Build history of the part. All positions in model axes, mm. Face numbers are marked on the shaded views. A direction names the side the tool comes from. Give positions to 0.01 mm unless a question says otherwise; leave off trailing zeros. Order: outer loops, then holes, each group sorted by start corner. A loop starts at its lowest first (then second) coordinate and runs counter-clockwise, first axis right, second up. Notation, with made-up numbers: (-0.75, 81) - (49.25, 81) arc R21 ccw to (49.25, 120) - close; hole circle Ø10 at (63, 63). An arc over 180 degrees is marked (long way). One line per item, written item: value.
```python
from build123d import *

# Parameters (mm, degrees)
F1_DEPTH = 50.8
F2_W     = 50.8
F2_H     = 127
F3_DEPTH = 76.2
F4_W     = 50.8
F4_H     = 25.4
F5_DEPTH = 25.4


with BuildPart() as f1:
    # F0 (on Front) → F1 (new body)
    with BuildSketch(Plane.XZ):
        Polygon((100.034788, 58.857108), (-103.165212, 58.857108), (-103.165212, -68.142892), (100.034788, -68.142892), (100.034788, -30.042892), (-1.565212, -30.042892), (-1.565212, 20.757108), (100.034788, 20.757108), align=None)
    extrude(amount=F1_DEPTH)

    # F2 (on face) → F3 (join)
    with BuildSketch(Plane(origin=(0, 0, 0), x_dir=(-1, 0, 0), z_dir=(0, 1, 0))):
        with Locations((77.765212, -4.642892)):
            Rectangle(F2_W, F2_H)
    extrude(amount=F3_DEPTH)

    # F4 (on face) → F5 (join)
    with BuildSketch(Plane(origin=(0, 76.2, 0), x_dir=(-1, 0, 0), z_dir=(0, 1, 0))):
        with Locations((77.765212, 46.157108)):
            Rectangle(F4_W, F4_H)
        with Locations((77.765212, -55.442892)):
            Rectangle(F4_W, F4_H)
    extrude(amount=F5_DEPTH)


solid = f1.part
```
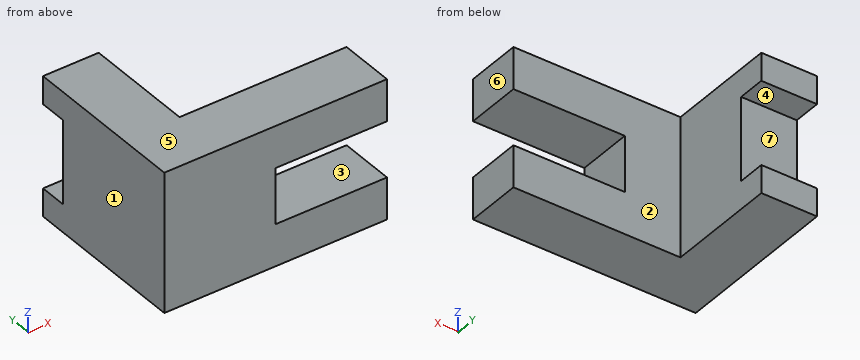
(1) Slice it at C-C, the plane z = -25. Give the cut face in (x, y), and give its area (3 significant figures).
Completed:
outline: (-103.17, -50.8) - (-1.57, -50.8) - (-1.57, 0) - (-52.37, 0) - (-52.37, 76.2) - (-103.17, 76.2) - close
area: 9,030 mm²
(2) Drill centre lines: line 1 (X direction, y = 1.5, z = -0.5); line 2 (Y direction, x = -22, z = 15); line 3 (X direction, y = -11.5, z = -8.5). Where is each one in solid material? Low to high.
Completed:
line 1: -103.17 to -52.37
line 2: -50.8 to 0
line 3: -103.17 to -1.57
(3) Slice it at A-A, the plane y = 89.5. Give the cut face in (x, z), and give its area (3 significant figures).
Completed:
outline: (-103.17, -68.14) - (-52.37, -68.14) - (-52.37, -42.74) - (-103.17, -42.74) - close; (-103.17, 33.46) - (-52.37, 33.46) - (-52.37, 58.86) - (-103.17, 58.86) - close
area: 2,580 mm²
(4) Slice it at D-D, the plane y = -9. Give the cut face in (x, z), and give its area (3 significant figures).
Completed:
outline: (-103.17, -68.14) - (100.03, -68.14) - (100.03, -30.04) - (-1.57, -30.04) - (-1.57, 20.76) - (100.03, 20.76) - (100.03, 58.86) - (-103.17, 58.86) - close
area: 20,600 mm²
(5) Slice it at B-B, the plane x = 1.5. Give the cut face in (y, z).
Completed:
outline: (-50.8, -68.14) - (0, -68.14) - (0, -30.04) - (-50.8, -30.04) - close; (-50.8, 20.76) - (0, 20.76) - (0, 58.86) - (-50.8, 58.86) - close
(6) 3-axis set-ups, long thin cutter, end or side, ignore diameter. For the marked faces 1, 2, 3 and 4: which of +Z, -Z, +X, -X, +Y, -Y reach the whole face in a straight line?
Completed:
face 1: +Z, -Z, -X, +Y, -Y
face 2: +Z, -Z, +X, +Y
face 3: +X, +Y, -Y
face 4: +X, -X, +Y
(7) Pull direction Z, two halves, no side cores. Call the marked faces 5, 6 and 7: +Z half, -Z half, draft (parallel to the pull), parting line (faces both ways), or undercut.
Completed:
face 5: +Z half
face 6: draft
face 7: undercut
(8) Pin check, flat tip, straight feed: P1, Ø1.5, axis at y = 71, z = -55, coming from the +X side. Stop position of the tip, or through.
Completed:
P1: x = -52.37
